Work out the finished part from the listing and answer in its coordinate system (mm). Face numbers are marked on the shaded views. A direction names the side the tool comes from. Coordinates: 2 decimals unless noted, no trailing zeros. Order: outer loops, then holes, each group sorted by start corner. A loop starts at its lowest first (then second) coordinate and runs counter-clockwise, first axis right, second up. Notation, with made-up numbers: M 57.25,-15 L 68.25,-15 A29 ccw 68.25,20 Z; hole C -17.75,40 d3. An arc over 180 degrees is marked long. Use a Markdown table: item, result.
from build123d import *

# Parameters (mm, degrees)
CROQUIS1_R              = 10
SALIENTE_EXTRUIR1_DEPTH = 2.5
CROQUIS2_R              = 4.5
SALIENTE_EXTRUIR2_DEPTH = 2
CROQUIS3_R              = 2.4
CORTAR_EXTRUIR1_DEPTH   = 15.84082208
CROQUIS4_R              = 1.25
CORTAR_EXTRUIR2_DEPTH   = 15.84082208


with BuildPart() as part:
    # Croquis1 → Saliente-Extruir1 (new body)
    with BuildSketch(Plane.XY):
        Circle(CROQUIS1_R)
    extrude(amount=SALIENTE_EXTRUIR1_DEPTH)

    # Croquis2 → Saliente-Extruir2 (add)
    with BuildSketch(Plane.XY.offset(2.5)):
        Circle(CROQUIS2_R)
    extrude(amount=SALIENTE_EXTRUIR2_DEPTH)

    # Croquis3 → Cortar-Extruir1 (cut, through all)
    with BuildSketch(Plane.XY.offset(4.5)):
        Circle(CROQUIS3_R)
    extrude(amount=-CORTAR_EXTRUIR1_DEPTH, mode=Mode.SUBTRACT)

    # Croquis4 → Cortar-Extruir2 (cut, through all)
    with BuildSketch(Plane(origin=(0, 0, 0), x_dir=(-1, 0, 0), z_dir=(0, 0, -1))):
        with Locations((0, 7)):
            Circle(CROQUIS4_R)
        with Locations((7, 0)):
            Circle(CROQUIS4_R)
        with Locations((0, -7)):
            Circle(CROQUIS4_R)
        with Locations((-7, 0)):
            Circle(CROQUIS4_R)
    extrude(amount=-CORTAR_EXTRUIR2_DEPTH, mode=Mode.SUBTRACT)


solid = part.part
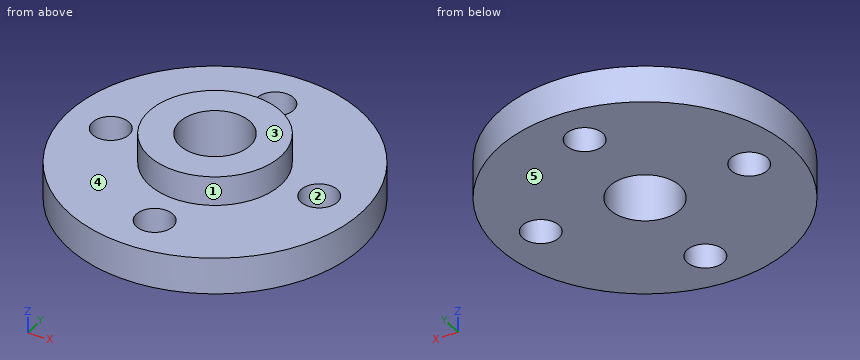
(1) Determine the mould class of the marked faces 1, 2 and 3 for opening direction Y: pulls with the +Y half, pulls with the -Y half, needs draft (parallel to the pull), parting line crosses it, or undercut.
Conclusion:
| item | result |
|---|---|
| face 1 | parting line crosses it |
| face 2 | undercut |
| face 3 | needs draft |
(2) Which of the six approach directions +Z, -Z, +X, -X, +Y, -Y give full straight-line access (tool end or side, diameter ignored) to the marked faces 4 and 5?
Conclusion:
| item | result |
|---|---|
| face 4 | +Z |
| face 5 | -Z, +X, -X, +Y, -Y |
(3) A cutting plane is placed at C-C (y = 2). Determine the outline of the cut face in (x, z).
Conclusion:
| item | result |
|---|---|
| outline | M -9.8,0 L -1.33,0 L -1.33,4.5 L -4.03,4.5 L -4.03,2.5 L -9.8,2.5 Z; M 1.33,0 L 9.8,0 L 9.8,2.5 L 4.03,2.5 L 4.03,4.5 L 1.33,4.5 Z |
(4) A cutting plane is placed at D-D (z = 0.7). Determine the outline of the cut face in (x, y).
Conclusion:
| item | result |
|---|---|
| outline | C 0,0 d20; hole C -7,0 d2.5; hole C 0,0 d4.8; hole C 0,-7 d2.5; hole C 0,7 d2.5; hole C 7,0 d2.5 |
(5) Given P1, Ø4, axis at x = 0, y = 7, coming from the +Z side, flat-ended and moving along its own axis, determine where the tip first touches the part or whether it passes through.
Conclusion:
| item | result |
|---|---|
| P1 | z = 2.5 |
(6) A cutting plane is placed at A-A (x = 6). Determine the outline of the cut face in (y, z).
Conclusion:
| item | result |
|---|---|
| outline | M -8,0 L -0.75,0 L -0.75,2.5 L -8,2.5 Z; M 0.75,0 L 8,0 L 8,2.5 L 0.75,2.5 Z |
(7) Straight lines are drawn through the part: L1, parallel to Y at x = 0, z = 1.75; L2, parallel to Y at x = -0.5, z = 0.95; L3, parallel to Z at x = -4, y = 8. For each, find the intervals that lie inside material, in ascending order.
Conclusion:
| item | result |
|---|---|
| L1 | -10 to -8.25, -5.75 to -2.4, 2.4 to 5.75, 8.25 to 10 |
| L2 | -9.99 to -8.15, -5.85 to -2.35, 2.35 to 5.85, 8.15 to 9.99 |
| L3 | 0 to 2.5 |
(8) A cutting plane is placed at B-B (x = 0). Determine the outline of the cut face in (y, z).
Conclusion:
| item | result |
|---|---|
| outline | M -10,0 L -8.25,0 L -8.25,2.5 L -10,2.5 Z; M -5.75,0 L -2.4,0 L -2.4,4.5 L -4.5,4.5 L -4.5,2.5 L -5.75,2.5 Z; M 2.4,0 L 5.75,0 L 5.75,2.5 L 4.5,2.5 L 4.5,4.5 L 2.4,4.5 Z; M 8.25,0 L 10,0 L 10,2.5 L 8.25,2.5 Z |
